from build123d import *

# Parameters (mm, degrees)
SKETCH1_W               = 25.4
SKETCH1_H               = 50.8
SKETCH1_W_2             = 19.05
SKETCH1_H_2             = 44.45
BOSS_EXTRUDE1_DEPTH     = 342.9
CUT_EXTRUDE1_DEPTH      = 1
CUT_EXTRUDE1_DEPTH_BACK = 26.4


with BuildPart() as part:
    # Sketch1 → Boss-Extrude1 (new body, symmetric)
    with BuildSketch(Plane(origin=(0, 0, 0), x_dir=(0, 0, -1), z_dir=(1, 0, 0))):
        Rectangle(SKETCH1_W, SKETCH1_H)
        Rectangle(SKETCH1_W_2, SKETCH1_H_2, mode=Mode.SUBTRACT)
    extrude(amount=BOSS_EXTRUDE1_DEPTH, both=True)

    # Sketch2 → Cut-Extrude1 (cut, two sides)
    with BuildSketch(Plane(origin=(0, 0, -12.7), x_dir=(-1, 0, 0), z_dir=(0, 0, -1))) as cut_extrude1_sk:
        Polygon((342.9, -25.4), (342.9, 25.4), (313.570606325, -25.4), align=None)
        Polygon((-342.9, -25.4), (-313.570606325, -25.4), (-342.9, 25.4), align=None)
    extrude(amount=CUT_EXTRUDE1_DEPTH, mode=Mode.SUBTRACT)
    extrude(cut_extrude1_sk.sketch, amount=-CUT_EXTRUDE1_DEPTH_BACK, mode=Mode.SUBTRACT)


solid = part.part
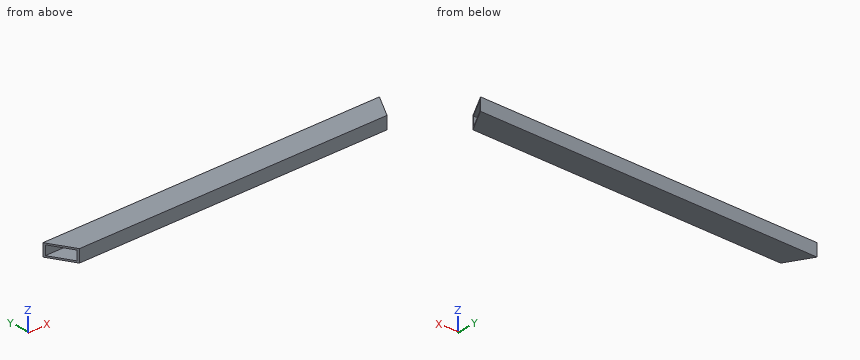
The model under review builds one solid part; all positions refer to its coordinate system, in mm. Give positions to 0.01 mm unless a question says otherwise; leave off trailing zeros. Write each loop counter-clockwise with the first axis right and the second up, starting at its lowest first coordinate (ties: lowest second). Pieces come first, ordered by that corner, then holes.
1. Add section A-A, the plane z = -1. Write out the cut boundary in (x, y) (3 decimals).
2. Wall thickness on L1, parallel to Z at x = 66, y = -16 (3 decimals); L2, parallel to Y at x = -216.5, z = -3.25 (3 decimals); L3, parallel to X at y = 22, z = 10: over which ranges is each line inside the solid? List them lowest first.
3. Add section C-C, the plane x = 101. Write out the cut boundary in (y, z) (3 decimals).
4. For P1, Ø6, axis at y = 12.5, z = -9.5, coming from the -X side, flat-tipped, find the tip position at first contact; note if it passes through.
5. Add section B-B, the plane y = -3. Write out the cut boundary in (x, z) (3 decimals).
Worked answers:
1. outline: (-342.9, 25.4) - (-341.067, 22.225) - (341.067, 22.225) - (342.9, 25.4) - close; (-315.404, -22.225) - (-313.571, -25.4) - (313.571, -25.4) - (315.404, -22.225) - close
2. L1: z = -12.7 to -9.525, 9.525 to 12.7
2. L2: y = -25.4 to -22.225, 22.225 to 25.4
2. L3: x = -340.94 to 340.94
3. outline: (-25.4, -12.7) - (25.4, -12.7) - (25.4, 12.7) - (-25.4, 12.7) - close; hole (-22.225, -9.525) - (22.225, -9.525) - (22.225, 9.525) - (-22.225, 9.525) - close
4. P1: stops at x = -337.18
5. outline: (-326.503, -12.7) - (326.503, -12.7) - (326.503, -9.525) - (-326.503, -9.525) - close; (-326.503, 9.525) - (326.503, 9.525) - (326.503, 12.7) - (-326.503, 12.7) - close
